Part model, mm, in its own coordinate system. Face numbers are marked on the shaded views. A direction names the side the tool comes from. Round coordinates to 2 decimals unless told otherwise and drop trailing zeros. Loops run counter-clockwise (first coordinate to the right, second up) from the corner with the lowest first, then second, coordinate; pieces in that order, holes last. Notation, with made-up numbers: M 24,64 L 68,64 A20 cw 68,86 Z; hole C 41.25,0.5 d2. An arc over 180 degrees is marked long. Write each question's results on one line, items separated by ' | '.
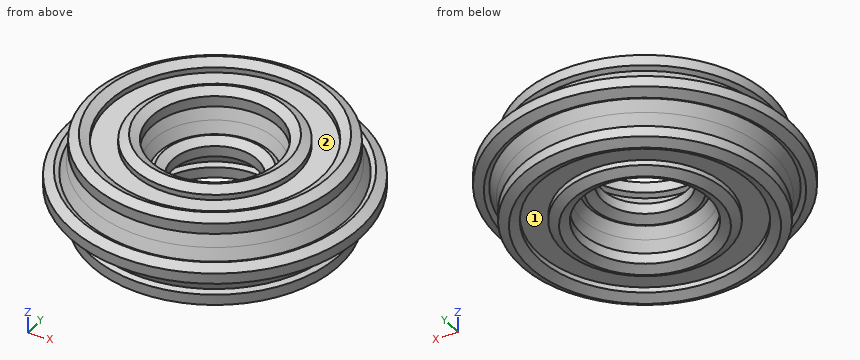
from build123d import *


with BuildPart() as f1:
    # F0 (on Front) → F1 (revolve)
    with BuildSketch(Plane.XZ):
        with BuildLine():
            ThreePointArc((-9.1840260647, 20.0261379157), (-8.8870457607, 17.9573039236), (-8.7877535299, 15.8696228078))
            ThreePointArc((-8.7877535299, 15.8696228078), (-8.8870457607, 13.7819416921), (-9.1840260647, 11.7131076999))
            Line((-9.1840260647, 11.7131076999), (-8.1344294431, 11.1071228078))
            Line((-8.1344294431, 11.1071228078), (-5.384798786, 15.8696228078))
            Line((-5.384798786, 15.8696228078), (-8.1344294431, 20.6321228078))
            Line((-8.1344294431, 20.6321228078), (-9.1840260647, 20.0261379157))
        make_face()
        with BuildLine():
            Line((-10.8840601001, 19.0446228078), (-9.1840260647, 20.0261379157))
            ThreePointArc((-9.1840260647, 20.0261379157), (-10.1735252451, 23.5537234722), (-11.7347988177, 26.8681454908))
            ThreePointArc((-11.7347988177, 26.8681454908), (-13.8245356754, 29.8774590153), (-16.3847647507, 32.4981831719))
            Line((-16.3847647507, 32.4981831719), (-18.084798786, 31.5166680639))
            Line((-18.084798786, 31.5166680639), (-23.5840601001, 34.6916680639))
            Line((-23.5840601001, 34.6916680639), (-23.5840601001, 36.6546982798))
            ThreePointArc((-23.5840601001, 36.6546982798), (-27.1337883649, 37.5615596255), (-30.784798786, 37.8666680639))
            ThreePointArc((-30.784798786, 37.8666680639), (-34.4358092072, 37.5615596255), (-37.985537472, 36.6546982798))
            Line((-37.985537472, 36.6546982798), (-37.985537472, 34.6916680639))
            Line((-37.985537472, 34.6916680639), (-43.484798786, 31.5166680639))
            Line((-43.484798786, 31.5166680639), (-45.1848328214, 32.4981831719))
            ThreePointArc((-45.1848328214, 32.4981831719), (-47.7450618967, 29.8774590153), (-49.8347987544, 26.8681454908))
            ThreePointArc((-49.8347987544, 26.8681454908), (-51.396072327, 23.5537234722), (-52.3855715074, 20.0261379157))
            Line((-52.3855715074, 20.0261379157), (-50.685537472, 19.0446228078))
            Line((-50.685537472, 19.0446228078), (-50.685537472, 12.6946228078))
            Line((-50.685537472, 12.6946228078), (-52.3855715074, 11.7131076999))
            ThreePointArc((-52.3855715074, 11.7131076999), (-51.3960723856, 8.1855223005), (-49.834798922, 4.8711004152))
            ThreePointArc((-49.834798922, 4.8711004152), (-47.7450620035, 1.8617867296), (-45.1848328214, -0.7589375563))
            Line((-45.1848328214, -0.7589375563), (-43.484798786, 0.2225775517))
            Line((-43.484798786, 0.2225775517), (-37.985537472, -2.9524224483))
            Line((-37.985537472, -2.9524224483), (-37.985537472, -4.9154526642))
            ThreePointArc((-37.985537472, -4.9154526642), (-34.4358092072, -5.8223140099), (-30.784798786, -6.1274224483))
            ThreePointArc((-30.784798786, -6.1274224483), (-27.1337883649, -5.8223140099), (-23.5840601001, -4.9154526642))
            Line((-23.5840601001, -4.9154526642), (-23.5840601001, -2.9524224483))
            Line((-23.5840601001, -2.9524224483), (-18.084798786, 0.2225775517))
            Line((-18.084798786, 0.2225775517), (-16.3847647507, -0.7589375563))
            ThreePointArc((-16.3847647507, -0.7589375563), (-13.8245356346, 1.8617866497), (-11.7347987537, 4.8711002358))
            ThreePointArc((-11.7347987537, 4.8711002358), (-10.1735252227, 8.1855222034), (-9.1840260647, 11.7131076999))
            Line((-9.1840260647, 11.7131076999), (-10.8840601001, 12.6946228078))
            Line((-10.8840601001, 12.6946228078), (-10.8840601001, 19.0446228078))
        make_face()
        with BuildLine():
            ThreePointArc((-11.7347988177, 26.8681454908), (-10.1735252451, 23.5537234722), (-9.1840260647, 20.0261379157))
            Line((-9.1840260647, 20.0261379157), (-8.1344294431, 20.6321228078))
            Line((-8.1344294431, 20.6321228078), (-11.7347988177, 26.8681454908))
        make_face()
        with BuildLine():
            Line((-8.1344294431, 11.1071228078), (-9.1840260647, 11.7131076999))
            ThreePointArc((-9.1840260647, 11.7131076999), (-10.1735252227, 8.1855222034), (-11.7347987537, 4.8711002358))
            Line((-11.7347987537, 4.8711002358), (-8.1344294431, 11.1071228078))
        make_face()
        with BuildLine():
            ThreePointArc((-16.3847647507, 32.4981831719), (-13.8245356754, 29.8774590153), (-11.7347988177, 26.8681454908))
            Line((-11.7347988177, 26.8681454908), (-15.335168129, 33.1041680639))
            Line((-15.335168129, 33.1041680639), (-16.3847647507, 32.4981831719))
        make_face()
        Polygon((-5.384798786, 22.2196228078), (-8.1344294431, 20.6321228078), (-5.384798786, 15.8696228078), (-8.1344294431, 11.1071228078), (-5.384798786, 9.5196228078), (0.114462528, 12.6946228078), (0.114462528, 19.0446228078), align=None)
        with BuildLine():
            Line((-15.335168129, -1.3649224483), (-11.7347987537, 4.8711002358))
            ThreePointArc((-11.7347987537, 4.8711002358), (-13.8245356346, 1.8617866497), (-16.3847647507, -0.7589375563))
            Line((-16.3847647507, -0.7589375563), (-15.335168129, -1.3649224483))
        make_face()
        with BuildLine():
            ThreePointArc((-23.5840601001, 36.6546982798), (-19.786276158, 34.9196228078), (-16.3847647507, 32.4981831719))
            Line((-16.3847647507, 32.4981831719), (-15.335168129, 33.1041680639))
            Line((-15.335168129, 33.1041680639), (-18.084798786, 37.8666680639))
            Line((-18.084798786, 37.8666680639), (-23.5840601001, 37.8666680639))
            Line((-23.5840601001, 37.8666680639), (-23.5840601001, 36.6546982798))
        make_face()
        Polygon((-18.084798786, 37.8666680639), (-15.335168129, 33.1041680639), (-12.585537472, 34.6916680639), (-12.585537472, 41.0416680639), (-18.084798786, 44.2166680639), (-23.5840601001, 41.0416680639), (-23.5840601001, 37.8666680639), align=None)
        with BuildLine():
            Line((-15.335168129, -1.3649224483), (-16.3847647507, -0.7589375563))
            ThreePointArc((-16.3847647507, -0.7589375563), (-19.786276158, -3.1803771922), (-23.5840601001, -4.9154526642))
            Line((-23.5840601001, -4.9154526642), (-23.5840601001, -6.1274224483))
            Line((-23.5840601001, -6.1274224483), (-18.084798786, -6.1274224483))
            Line((-18.084798786, -6.1274224483), (-15.335168129, -1.3649224483))
        make_face()
        Polygon((-12.585537472, -2.9524224483), (-15.335168129, -1.3649224483), (-18.084798786, -6.1274224483), (-23.5840601001, -6.1274224483), (-23.5840601001, -9.3024224483), (-18.084798786, -12.4774224483), (-12.585537472, -9.3024224483), align=None)
        with BuildLine():
            ThreePointArc((-30.784798786, 37.8666680639), (-27.1337883649, 37.5615596255), (-23.5840601001, 36.6546982798))
            Line((-23.5840601001, 36.6546982798), (-23.5840601001, 37.8666680639))
            Line((-23.5840601001, 37.8666680639), (-30.784798786, 37.8666680639))
        make_face()
        with BuildLine():
            Line((-23.5840601001, -6.1274224483), (-23.5840601001, -4.9154526642))
            ThreePointArc((-23.5840601001, -4.9154526642), (-27.1337883649, -5.8223140099), (-30.784798786, -6.1274224483))
            Line((-30.784798786, -6.1274224483), (-23.5840601001, -6.1274224483))
        make_face()
        with BuildLine():
            ThreePointArc((-37.985537472, 36.6546982798), (-34.4358092072, 37.5615596255), (-30.784798786, 37.8666680639))
            Line((-30.784798786, 37.8666680639), (-37.985537472, 37.8666680639))
            Line((-37.985537472, 37.8666680639), (-37.985537472, 36.6546982798))
        make_face()
        with BuildLine():
            Line((-37.985537472, -6.1274224483), (-30.784798786, -6.1274224483))
            ThreePointArc((-30.784798786, -6.1274224483), (-34.4358092072, -5.8223140099), (-37.985537472, -4.9154526642))
            Line((-37.985537472, -4.9154526642), (-37.985537472, -6.1274224483))
        make_face()
        with BuildLine():
            ThreePointArc((-45.1848328214, 32.4981831719), (-41.7833214141, 34.9196228078), (-37.985537472, 36.6546982798))
            Line((-37.985537472, 36.6546982798), (-37.985537472, 37.8666680639))
            Line((-37.985537472, 37.8666680639), (-43.484798786, 37.8666680639))
            Line((-43.484798786, 37.8666680639), (-46.2344294431, 33.1041680639))
            Line((-46.2344294431, 33.1041680639), (-45.1848328214, 32.4981831719))
        make_face()
        Polygon((-43.484798786, 37.8666680639), (-37.985537472, 37.8666680639), (-37.985537472, 41.0416680639), (-43.484798786, 44.2166680639), (-48.9840601001, 41.0416680639), (-48.9840601001, 34.6916680639), (-46.2344294431, 33.1041680639), align=None)
        with BuildLine():
            Line((-37.985537472, -6.1274224483), (-37.985537472, -4.9154526642))
            ThreePointArc((-37.985537472, -4.9154526642), (-41.7833214141, -3.1803771922), (-45.1848328214, -0.7589375563))
            Line((-45.1848328214, -0.7589375563), (-46.2344294431, -1.3649224483))
            Line((-46.2344294431, -1.3649224483), (-43.484798786, -6.1274224483))
            Line((-43.484798786, -6.1274224483), (-37.985537472, -6.1274224483))
        make_face()
        Polygon((-37.985537472, -9.3024224483), (-37.985537472, -6.1274224483), (-43.484798786, -6.1274224483), (-46.2344294431, -1.3649224483), (-48.9840601001, -2.9524224483), (-48.9840601001, -9.3024224483), (-43.484798786, -12.4774224483), align=None)
        with BuildLine():
            ThreePointArc((-49.8347987544, 26.8681454908), (-47.7450618967, 29.8774590153), (-45.1848328214, 32.4981831719))
            Line((-45.1848328214, 32.4981831719), (-46.2344294431, 33.1041680639))
            Line((-46.2344294431, 33.1041680639), (-49.8347987544, 26.8681454908))
        make_face()
        with BuildLine():
            Line((-46.2344294431, -1.3649224483), (-45.1848328214, -0.7589375563))
            ThreePointArc((-45.1848328214, -0.7589375563), (-47.7450620035, 1.8617867296), (-49.834798922, 4.8711004152))
            Line((-49.834798922, 4.8711004152), (-46.2344294431, -1.3649224483))
        make_face()
        with BuildLine():
            ThreePointArc((-52.3855715074, 20.0261379157), (-51.396072327, 23.5537234722), (-49.8347987544, 26.8681454908))
            Line((-49.8347987544, 26.8681454908), (-53.435168129, 20.6321228078))
            Line((-53.435168129, 20.6321228078), (-52.3855715074, 20.0261379157))
        make_face()
        with BuildLine():
            Line((-53.435168129, 11.1071228078), (-49.834798922, 4.8711004152))
            ThreePointArc((-49.834798922, 4.8711004152), (-51.3960723856, 8.1855223005), (-52.3855715074, 11.7131076999))
            Line((-52.3855715074, 11.7131076999), (-53.435168129, 11.1071228078))
        make_face()
        with BuildLine():
            ThreePointArc((-52.3855715074, 11.7131076999), (-52.7818440422, 15.8696228078), (-52.3855715074, 20.0261379157))
            Line((-52.3855715074, 20.0261379157), (-53.435168129, 20.6321228078))
            Line((-53.435168129, 20.6321228078), (-56.184798786, 15.8696228078))
            Line((-56.184798786, 15.8696228078), (-53.435168129, 11.1071228078))
            Line((-53.435168129, 11.1071228078), (-52.3855715074, 11.7131076999))
        make_face()
        Polygon((-56.184798786, 15.8696228078), (-53.435168129, 20.6321228078), (-56.184798786, 22.2196228078), (-61.6840601001, 19.0446228078), (-61.6840601001, 12.6946228078), (-56.184798786, 9.5196228078), (-53.435168129, 11.1071228078), align=None)
    revolve(axis=Axis((25.514462528, 0, 17.1541441232), (0, 0, -1)))


solid = f1.part
Item 1: Band-saw the part on A-A on x = 42. Count the separate pieces of the cut face and the enclosed holes in it, and give its area (3 significant figures).
Filled sheet:
separate pieces: 2 | enclosed holes: 12 | area: 4,250 mm^2
Item 2: Wall check: L1, parallel to Z at x = -19.5, y = 19; L2, parallel to X at y = 7, z = 39.5; L3, parallel to Y at x = 64, z = 19.5. Give the ranges that are in metal, low to high.
Filled sheet:
L1: -9.44 to -4.83, -2.81 to 34.55, 36.57 to 41.18 | L2: -48.65 to -37.6, -23.08 to -11.94, 62.97 to 74.11, 88.63 to 99.68 | L3: -77.37 to -67.84, -66.68 to 66.68, 67.84 to 77.37
Item 3: Drop flat-ended pins along their axis: P1, Ø2, axis at y = 48, z = 33.5, coming from the +X side; P2, Ø3, axis at x = -32, z = 13, coming from the -Y side; P3, Ø2, axis at x = 51, z = 34.5, coming from the -Y side. Give the stop position or say it passes through.
Filled sheet:
P1: x = 82.21 | P2: y = -66.83 | P3: y = -70.35
Item 4: Band-saw the part on B-B on z = 2.5. Give the cut face in (x, y).
Filled sheet:
outline: C 25.51,0 d147.96; hole C 25.51,0 d77.24
Item 5: Which spindle directions (+Z, -Z, +X, -X, +Y, -Y) get a long thin tool onto all of the face, cutting with end or side? Do the marked faces 1 and 2. Say none if no direction does.
Filled sheet:
face 1: -Z | face 2: +Z
